from build123d import *

# Parameters (mm, degrees)
ESQUISSE1_W        = 15.24
ESQUISSE1_H        = 16.51
ESQUISSE1_R        = 1.5
PCB_DEPTH          = 1.4
ESQUISSE2_W        = 3
ESQUISSE2_H        = 5
ADXL345_DEPTH      = 0.8
ESQUISSE3_W        = 4
ESQUISSE3_H        = 4
ITG_3200_DEPTH     = 0.8
ESQUISSE6_R        = 0.5
BOSS_EXTRU_9_DEPTH = 7.4


with BuildPart() as part:
    # Esquisse1 → PCB (new body)
    with BuildSketch(Plane(origin=(0, 0, 0), x_dir=(1, 0, 0), z_dir=(0, 1, 0))):
        with Locations((-0.009586777, 2.926831956)):
            Rectangle(ESQUISSE1_W, ESQUISSE1_H)
        with Locations(Location((-5.089586777, 8.641831956, 0), (0, 0, 270))):
            Circle(ESQUISSE1_R, mode=Mode.SUBTRACT)
        with Locations(Location((5.070413223, 8.641831956, 0), (0, 0, 270))):
            Circle(ESQUISSE1_R, mode=Mode.SUBTRACT)
    extrude(amount=PCB_DEPTH)

    # Esquisse2 → ADXL345 (add)
    with BuildSketch(Plane(origin=(0, 1.4, 0), x_dir=(1, 0, 0), z_dir=(0, 1, 0))):
        with Locations((-3.819586777, 1.021831956)):
            Rectangle(ESQUISSE2_W, ESQUISSE2_H)
    extrude(amount=ADXL345_DEPTH)

    # Esquisse3 → ITG-3200 (add)
    with BuildSketch(Plane(origin=(0, 1.4, 0), x_dir=(1, 0, 0), z_dir=(0, 1, 0))):
        with Locations((2.530413223, 1.021831956)):
            Rectangle(ESQUISSE3_W, ESQUISSE3_H)
    extrude(amount=ITG_3200_DEPTH)

    # Esquisse6 → Boss.-Extru.9 (add)
    with BuildSketch(Plane.XZ):
        with Locations(Location((-6.359586777, 4.064307622, 0), (0, 0, 90))):
            Circle(ESQUISSE6_R)
        with Locations(Location((-3.819586777, 4.064307622, 0), (0, 0, 90))):
            Circle(ESQUISSE6_R)
        with Locations(Location((-1.279586777, 4.064307622, 0), (0, 0, 90))):
            Circle(ESQUISSE6_R)
        with Locations(Location((1.260413223, 4.064307622, 0), (0, 0, 90))):
            Circle(ESQUISSE6_R)
        with Locations(Location((3.800413223, 4.064307622, 0), (0, 0, 90))):
            Circle(ESQUISSE6_R)
        with Locations(Location((6.340413223, 4.064307622, 0), (0, 0, 90))):
            Circle(ESQUISSE6_R)
    extrude(amount=BOSS_EXTRU_9_DEPTH)


solid = part.part
Here's how the part is built. I have some questions about the finished solid (model axes, mm). A direction names the side the tool comes from. Give positions to 0.01 mm unless a question says otherwise; leave off trailing zeros. Order: outer loops, then holes, each group sorted by start corner. A loop starts at its lowest first (then second) coordinate and runs counter-clockwise, first axis right, second up. Notation, with made-up numbers: M 48,38 L 103,38 A22 cw 103,69 Z; hole C -9,20 d3. An arc over 180 degrees is marked long. Answer as a JSON object with one key per item and string values. Group by question number.
1) Suppose I cut it at B-B, the plane x = 3. Write out the boundary of the cut face in (y, z).
2) On a 3-axis mill with a long thin cutter (end or side, diameter ignored), from which of +Z, -Z, +X, -X, +Y, -Y can I reach the whole of each face in a straight line? I mean faces 1 (the flat face through (0.53, 2, -1)), 2 (the flat face through (3, 2, 0.978)), 3 (the cylindrical face through (-0.975, -3.648, 3.668)). Say none if no direction works.
3) We'd pull the mould along X, two halves only. Please class faces 4 (the cylindrical face through (-6.002, 0.69, -9.832)), 5 (the flat face through (4.53, 2, -1)), 6 (the flat face through (0, 1, -11.182)): pulls with the +X half, pulls with the -X half, needs draft (parallel to the pull), parting line crosses it, or undercut.
4) Suppose I cut it at A-A, the plane y = 1.75. Write out the boundary of the cut face in (x, z).
5) I'm going to push flat-ended pins straight in: pin 1 Ø5 at (x, z) = (5.07, -8.64) entering from -Y; pin 2 Ø0.9 at (y, z) = (1.5, -0.5) entering from -X; pin 3 Ø0.9 at (x, y) = (3.5, 2) entering from -Z; pin 4 Ø0.9 at (x, y) = (3, 2) entering from +Z. Where does each tip first touch, or does it pass through?
6) Suppose I cut it at C-C, the plane z = -9.75. Write out the boundary of the cut face in (x, y), plus the area to 3 significant figures.
7) Please list where these lines run through material, in increasing order: L1, parallel to Y at x = -4.75, z = -2.25; L2, parallel to Y at x = -2.25, z = -7.5; L3, parallel to Z at x = -3.75, y = -3.5. Write a range as [from, to].
8) Suppose I cut it at D-D, the plane z = -2.25. Write out the boundary of the cut face in (x, y).
Results found:
{
 "1": {"outline": "M 0,-11.18 L 1.4,-11.18 L 1.4,-3.02 L 2.2,-3.02 L 2.2,0.98 L 1.4,0.98 L 1.4,5.33 L 0,5.33 Z"},
 "2": {"face 1": "+Z, -Z, +Y", "face 2": "+Z, +X, +Y", "face 3": "-Y"},
 "3": {"face 4": "undercut", "face 5": "pulls with the +X half", "face 6": "needs draft"},
 "4": {"outline": "M -5.32,-3.52 L -2.32,-3.52 L -2.32,1.48 L -5.32,1.48 Z; M 0.53,-3.02 L 4.53,-3.02 L 4.53,0.98 L 0.53,0.98 Z"},
 "5": {"pin 1": "y = 0", "pin 2": "x = -7.63", "pin 3": "z = -3.02", "pin 4": "z = 0.98"},
 "6": {"outline": "M -7.63,0 L -6.1,0 L -6.1,1.4 L -7.63,1.4 Z; M -4.08,0 L 4.06,0 L 4.06,1.4 L -4.08,1.4 Z; M 6.08,0 L 7.61,0 L 7.61,1.4 L 6.08,1.4 Z", "area": "15.7 mm²"},
 "7": {"L1": "[0, 2.2]", "L2": "[0, 1.4]", "L3": "[3.57, 4.56]"},
 "8": {"outline": "M -7.63,0 L 7.61,0 L 7.61,1.4 L 4.53,1.4 L 4.53,2.2 L 0.53,2.2 L 0.53,1.4 L -2.32,1.4 L -2.32,2.2 L -5.32,2.2 L -5.32,1.4 L -7.63,1.4 Z"}
}
